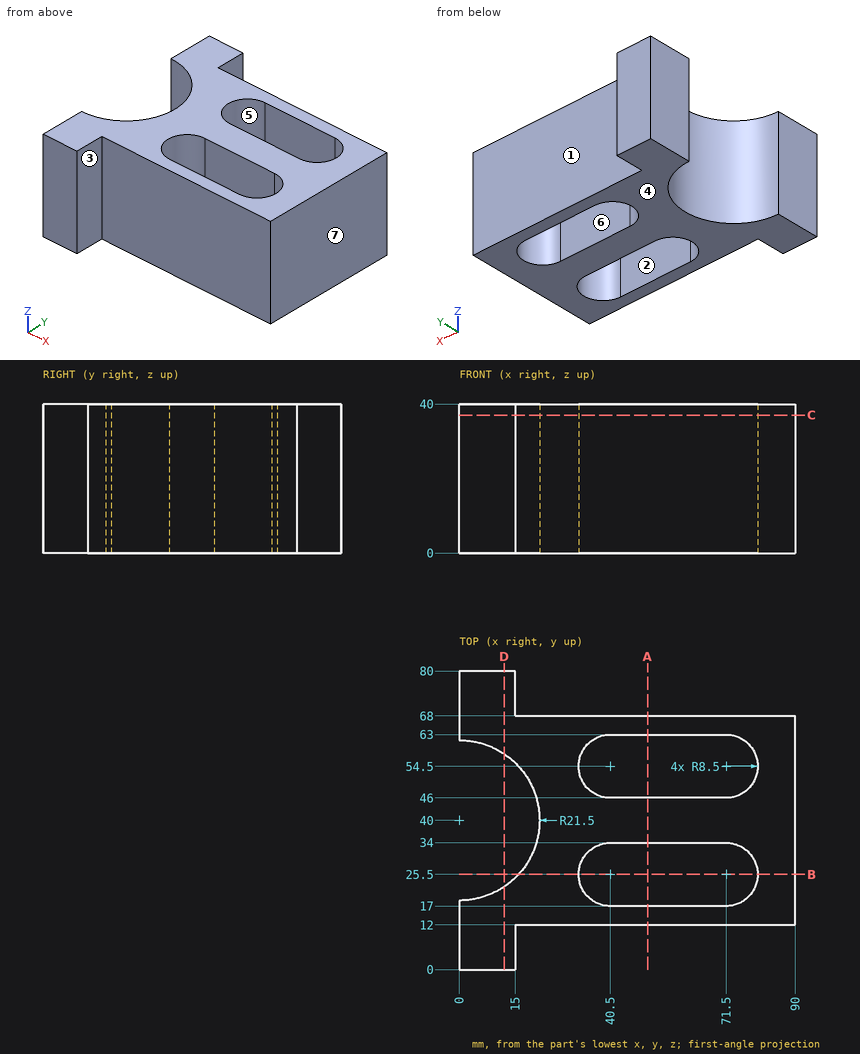
The drawing under review shows one solid part. Ordinate dimensions are in mm from its lowest x, y, z. A direction names the side the tool comes from. Coordinates: 2 decimals unless noted, no trailing zeros. Write each loop counter-clockwise with the first axis right and the second up, starting at its lowest first coordinate (ties: lowest second). Pieces come first, ordered by that corner, then holes.
1) Add section A-A (x = 50.5). Write out the cut boundary in (y, z).
2) Mouldability with a two-part tool opening along X and no side actions: class the marked faces 4, 5, 6 and 7 as +X half, -X half, draft (parallel to the pull), parting line (faces both ways), or undercut.
3) Add section D-D (x = 12). Write out the cut boundary in (y, z), plus the area to 3 significant figures.
4) Insertion check: pin 1 (3.5 mm diameter, centred on y = 73.5, z = 16.5, fed in from +X); pin 2 (3 mm diameter, centred on x = 72.5, z = 27, fed in from -Y); pin 3 (4 mm diameter, centred on x = 51, z = 36, fed in from +Y). Each pin has a flat end and moves straight along its axis. Give the tip position at first contact, or say it passes through.
5) To check wall thickness, follow L1, parallel to Y at x = 60.5, z = 37; L2, parallel to X at y = 59.5, z = 35; L3, parallel to Y at x = 19.5, z = 22. State the ranges of each line that lie inside material, in increasing order.
6) Add section C-C (z = 37). Write out the cut boundary in (x, y).
7) Machinability: for the marked faces 1, 2 and 3, which of the approach directions +Z, -Z, +X, -X, +Y, -Y give a long, thin tool a straight path to every point of the face, cutting with its end or side? Answer none if there is none.
8) Add section B-B (y = 25.5). Write out the cut boundary in (x, z).
Check result:
1. outline: (12, 0) - (17, 0) - (17, 40) - (12, 40) - close; (34, 0) - (46, 0) - (46, 40) - (34, 40) - close; (63, 0) - (68, 0) - (68, 40) - (63, 40) - close
2. face 4: draft
2. face 5: undercut
2. face 6: undercut
2. face 7: +X half
3. outline: (0, 0) - (22.16, 0) - (22.16, 40) - (0, 40) - close; (57.84, 0) - (80, 0) - (80, 40) - (57.84, 40) - close
3. area: 1,770 mm2
4. pin 1: stops at x = 15
4. pin 2: stops at y = 12
4. pin 3: stops at y = 68
5. L1: y = 12 to 17, 34 to 46, 63 to 68
5. L2: x = 9.06 to 33.63, 78.37 to 90
5. L3: y = 12 to 30.94, 49.06 to 68
6. outline: (0, 0) - (15, 0) - (15, 12) - (90, 12) - (90, 68) - (15, 68) - (15, 80) - (0, 80) - (0, 61.5) arc R21.5 cw to (0, 18.5) - close; hole (40.5, 17) - (71.5, 17) arc R8.5 ccw to (71.5, 34) - (40.5, 34) arc R8.5 ccw to start; hole (40.5, 46) - (71.5, 46) arc R8.5 ccw to (71.5, 63) - (40.5, 63) arc R8.5 ccw to start
7. face 1: +Z, -Z, +X, +Y
7. face 2: +Z, -Z
7. face 3: +Z, -Z, +X, -Y
8. outline: (15.87, 0) - (32, 0) - (32, 40) - (15.87, 40) - close; (80, 0) - (90, 0) - (90, 40) - (80, 40) - close
